from build123d import *

# Parameters (mm, degrees)
F1_DEPTH = 12.5
F3_DEPTH = 2.5
F4_R     = 1.983726
F5_R     = 4.05
F6_DEPTH = 12.5


with BuildPart() as f1:
    # F0 (on Front) → F1 (new body, symmetric)
    with BuildSketch(Plane.XZ):
        with BuildLine():
            Line((65, 0), (15, 0))
            Line((15, 0), (15, 44.3))
            Line((15, 44.3), (0, 44.3))
            Line((0, 44.3), (0, 39.3))
            Line((0, 39.3), (10, 39.3))
            Line((10, 39.3), (10, -5))
            Line((10, -5), (75, -5))
            Line((75, -5), (75, 50))
            ThreePointArc((75, 50), (70, 47.623014), (65, 50))
            Line((65, 50), (65, 0))
        make_face()
        with BuildLine():
            Line((75, 50), (65, 50))
            ThreePointArc((65, 50), (70, 47.623014), (75, 50))
        make_face()
        with BuildLine():
            ThreePointArc((76.447254, 54.070268), (67.840045, 60.144943), (65, 50))
            Line((65, 50), (75, 50))
            ThreePointArc((75, 50), (76.074675, 51.910313), (76.447254, 54.070268))
        make_face()
    extrude(amount=F1_DEPTH, both=True)

    # F2 (on Front) → F3 (join, symmetric)
    with BuildSketch(Plane.XZ):
        Polygon((15.042217, 15), (15.042217, 0), (30.042217, 0), align=None)
        Polygon((50, 0), (65, 0), (65, 15), align=None)
    extrude(amount=F3_DEPTH, both=True)

    # F4
    f4_edges = [f1.edges().sort_by_distance(p)[0] for p in [
        (15, 0, 44.3),
    ]]
    fillet(f4_edges, radius=F4_R)

    # F5 (on Front) → F6 (cut, through all)
    with BuildSketch(Plane.XZ):
        with Locations((70, 54.070268)):
            Circle(F5_R)
    extrude(amount=-F6_DEPTH, mode=Mode.SUBTRACT)

    # F7: F1 across plane


with BuildPart() as f1_1:
    add(f1.part)
    add(f1.part.mirror(Plane.YZ))


solid = f1_1.part
Work out the finished part from the listing and answer in its coordinate system (mm). A direction names the side the tool comes from. Give positions to 0.01 mm unless a question says otherwise; leave off trailing zeros. Loops run counter-clockwise (first coordinate to the right, second up) from the corner with the lowest first, then second, coordinate; pieces in that order, holes last. Notation, with made-up numbers: (29, -26.5) -> (58, -26.5) arc R23 cw to (58, -1.5) -> close; hole circle Ø8 at (84, -2). An arc over 180 degrees is marked (long way). Use a Markdown table: item, result. Add a question column.
1. Flat-ended cylindrical pins translate along their axes: pin 1 Ø5 at (x, y) = (-24, -6.5) entering from +Z; pin 2 Ø12 at (y, z) = (4.5, 34) entering from +X; pin 3 Ø12 at (x, z) = (23, 10) entering from -Y. Find the tip coordinate at first contact, or state that the pin passes through.
2. Section D-D on y = -6.25 is taken. Determine the outline of the cut face in (x, z), and give its area (3 significant figures).
3. Section A-A on y = 6.25 is taken. Determine the outline of the cut face in (x, z).
4. Section B-B on z = 6 is taken. State how many separate pieces and enclosed holes the cut face has, and give its area (3 significant figures).
5. Section C-C on z = 28.5 is taken. Determine the outline of the cut face in (x, y).
6. Determine the mould class of faces 4 (the flat face through (65, 0, 25)), 5 (the flat face through (0, 0, 39.3)), 6 (the flat face through (10, 0, 17)) for opening direction Z: released by +Z, released by -Z, zero draft, split by the parting line, or undercut.
7. Find the intervals of material crossed by probe 1 along X at (y, z) = (-8.75, 31.5); probe 2 along X at (y, z) = (7.75, 40); probe 3 along X at (y, z) = (11, 46), in increasing order.
8. For faces 1 (the flat face through (-19, -2.5, 4)), 2 (the flat face through (19, 2.5, 4)), 3 (the flat face through (-61, 2.5, 4)), determine the directions among +Z, -Z, +X, -X, +Y, -Y from which every point of the face is accessible in a straight line to the end or side of a thin tool.
Results below:
| question | item | result |
|---|---|---|
| 1 | pin 1 | stops at z = 0 |
| 1 | pin 2 | stops at x = 75 |
| 1 | pin 3 | stops at y = -2.5 |
| 2 | outline | (-76.45, 54.07) arc R6.45 ccw to (-75, 50) -> (-75, -5) -> (-10, -5) -> (-10, 39.3) -> (10, 39.3) -> (10, -5) -> (75, -5) -> (75, 50) arc R6.45 ccw to (76.45, 54.07) arc R6.45 ccw (long way) to (65, 50) -> (65, 0) -> (15, 0) -> (15, 42.32) arc R1.98 ccw to (13.02, 44.3) -> (-13.02, 44.3) arc R1.98 ccw to (-15, 42.32) -> (-15, 0) -> (-65, 0) -> (-65, 50) arc R6.45 ccw (long way) to start |
| 2 | area | 2,420 mm^2 |
| 3 | outline | (-76.45, 54.07) arc R6.45 ccw to (-75, 50) -> (-75, -5) -> (-10, -5) -> (-10, 39.3) -> (10, 39.3) -> (10, -5) -> (75, -5) -> (75, 50) arc R6.45 ccw to (76.45, 54.07) arc R6.45 ccw (long way) to (65, 50) -> (65, 0) -> (15, 0) -> (15, 42.32) arc R1.98 ccw to (13.02, 44.3) -> (-13.02, 44.3) arc R1.98 ccw to (-15, 42.32) -> (-15, 0) -> (-65, 0) -> (-65, 50) arc R6.45 ccw (long way) to start; hole circle Ø8.1 at (-70, 54.07); hole circle Ø8.1 at (70, 54.07) |
| 4 | separate pieces | 6 |
| 4 | enclosed holes | 0 |
| 4 | area | 930 mm^2 |
| 5 | outline | (-75, -12.5) -> (-65, -12.5) -> (-65, 12.5) -> (-75, 12.5) -> close; (-15, -12.5) -> (-10, -12.5) -> (-10, 12.5) -> (-15, 12.5) -> close; (10, -12.5) -> (15, -12.5) -> (15, 12.5) -> (10, 12.5) -> close; (65, -12.5) -> (75, -12.5) -> (75, 12.5) -> (65, 12.5) -> close |
| 6 | face 4 | undercut |
| 6 | face 5 | released by -Z |
| 6 | face 6 | zero draft |
| 7 | probe 1 | x = -75 to -65, -15 to -10, 10 to 15, 65 to 75 |
| 7 | probe 2 | x = -75 to -65, -15 to 15, 65 to 75 |
| 7 | probe 3 | x = -75 to -65, 65 to 75 |
| 8 | face 1 | +Z, -Y |
| 8 | face 2 | +Z, +Y |
| 8 | face 3 | +Y |
